Check sheet for the modelled part. Datum: model origin and axes. Units: mm. A direction names the side the tool comes from. Give positions to 0.01 mm unless a question says otherwise; leave off trailing zeros. Write each loop counter-clockwise with the first axis right and the second up, starting at its lowest first coordinate (ties: lowest second). Pieces come first, ordered by that corner, then holes. Notation, with made-up numbers: M 0.25,-2.75 L 16.25,-2.75 A6 cw 16.25,4.25 Z; hole C -27.75,-26 d5. An arc over 180 degrees is marked long. Write item = value, one per line. Start each with the question number.
1) Sectioned sample at D-D, the plane x = -0.5. Record the cut outline in (y, z), then the cut area to 3 significant figures.
2) Scan lines: L1, parallel to X at y = 3.5, z = -1.9; L2, parallel to Y at x = 3.5, z = 1.1; L3, parallel to X at y = -4.5, z = 1.75. Record each from-to range of solid material in increasing order.
3) Sectioned sample at B-B, the plane y = -3.75. Record the cut outline in (x, z), then the cut area to 3 significant figures.
4) Gauge pin test, flat ends, axial feed: pin 1 (0.5 mm diameter, centred on x = -2.5, z = 0.5, fed in from -Y); pin 2 (1.6 mm diameter, centred on x = -1.5, z = 1, fed in from +Y). Record the tip position at first contact, or that the pin passes through.
5) Sectioned sample at A-A, the plane x = 3.5. Record the cut outline in (y, z).
6) Sectioned sample at C-C, the plane z = 2.1. Record the cut outline in (x, y), then the cut area to 3 significant figures.
7) Draft check along X on faces 1 (the face through (5, -4, 0)), 2 (the face through (2, -7, 0)), 3 (the face through (0, 5, 0)), 4 (the face through (-3, 0, 0)). Enter one of: pulls with the +X half, pulls with the -X half, needs draft (parallel to the pull), parting line crosses it, or undercut.
8) Set-up check for faces 5 (the face through (-2.5, 4, 0)), 6 (the face through (-0.986, 2.048, -1.984)), 7 (the face through (-2.5, -4, 0)), 8 (the face through (4, -1, 0)): record each of +Z, -Z, +X, -X, +Y, -Y from which the full face is reachable in a straight line by a thin tool's end or side.
Autodesk Fusion 360 part; units mm, degrees
ref_plane "WorkPlane1" through (11.25, 0, 0) normal (1, 0, 0) x (0, 1, 0)
sketch "wire_screw2" plane through (0, 0, 0) normal (1, 0, 0) x (0, 1, 0)
  line L0 (7, 3.1) -> (-7, -3.1) construction
  line L1 (-7, 3.1) -> (7, -3.1) construction
  line L2 (-4, 4) -> (-4, -3.4897)
  line L3 (4, 4) -> (4, -3.5621)
  circle A0 centre (0, 0) radius 3.1
  circle A1 centre (0, 0) radius 2.75
  line L4 (-3.0288, -3.6864) -> (-3.0994, -0.0604)
  arc A2 (0, 2.75) -> (-3.0994, -0.0604) centre (0, -0.3643) ccw
  arc A3 (0, -2.75) -> (0, 2.75) centre (0, 0) ccw
  arc A4 (0, -2.75) -> (3.1, 0) centre (0, 0.3723) ccw
  line L5 (3.1, 0) -> (3.1, 3.8294)
  line L6 (0, 2.75) -> (3.1, 2.75)
  line L7 (0, -2.75) -> (-3.047, -2.75)
  line L8 (0, 2.75) -> (7, 2.75)
  line L9 (7, 2.75) -> (-7, 2.75)
  line L10 (-7, 2.75) -> (-7, -2.75)
  line L11 (-7, -2.75) -> (7, -2.75)
  line L12 (7, -2.75) -> (7, 2.75)
  dimension "d38" = 14
  dimension "d39" = 6.2
  dimension "d40" = 5.5
  dimension "d41" = 7
  dimension "d42" = 14
extrude "Extrude7" add sketch "wire_screw2" along normal blind -2 and the other way blind 3 contours L2 A0 L4 L9 L11 | A0 A2 L9 | A0 L4 L7 L11 | A0 L5 L6 L8 L9 | A0 A1 A3 A4 L6 L8 L9 | A0 A1 A2 L7 L11 | A1 A3 | L3 A0 L5 L8 L9 L11 | A0 A4 L11
extrude "Extrude8" add sketch "wire_screw2" against normal blind 2 contours A0 L4 L7 L11 | A0 L5 L6 L8 L9 | A0 A1 A3 A4 L6 L8 L9 | A0 A1 A2 L7 L11 | A1 A3
extrude "Extrude9" add sketch "wire_screw2" along normal blind 5 contours L2 A0 L4 L9 L11 | L2 L9 L10 L11 | A0 A2 L9 | A0 L4 L7 L11 | A0 L5 L6 L8 L9 | A0 A1 A3 A4 L6 L8 L9 | A0 A1 A2 L7 L11 | A1 A3 | L3 A0 L5 L8 L9 L11 | A0 A4 L11 | L3 L8 L9 L11 L12
sketch "wire_screw2_slot" plane through (0, 0, -2.75) normal (0, 0, -1) x (1, 0, 0)
  line L0 (-2, -4) -> (-2, 0)
  line L1 (-2, 0) -> (0, 0)
  line L2 (0, 0) -> (0, -7)
  line L3 (0, -7) -> (5, -7)
  line L4 (5, -7) -> (5, 7)
  line L5 (5, 7) -> (0, 7)
  line L6 (0, 7) -> (0, 3.047)
  line L7 (0, 3.047) -> (-2, 3.047)
  line L8 (-2, 3.047) -> (-2, 4)
  line L9 (-2, 4) -> (-3, 4)
  line L10 (-3, 4) -> (-3, -4)
  line L11 (-3, -4) -> (-2, -4)
  line L12 (3, 1) -> (7, 1)
  line L13 (7, 1) -> (7, -1)
  line L14 (7, -1) -> (3, -1)
  line L15 (3, -1) -> (3, 1)
  line L16 (3, 1) -> (7, -1) construction
  line L17 (7, 1) -> (3, -1) construction
  point P0 (5, 0)
  dimension "d51" = 4
  dimension "d52" = 2
extrude "Extrude10" cut sketch "wire_screw2_slot" against normal blind 8 contours L4 L12 L14 L15
Data:
q1.outline = M -3.1,-0.06 L -3.05,-2.75 L 0,-2.75 A3.12 ccw 3.1,0 L 3.1,2.75 L 0,2.75 A3.11 ccw Z
q1.area = 30.0 mm2
q2.L1 = -3 to -2, 0 to 5
q2.L2 = -7 to -1, 1 to 7
q2.L3 = 0 to 5
q3.outline = M -3,-2.75 L -2,-2.75 L -2,2.75 L -3,2.75 Z; M 0,-2.75 L 5,-2.75 L 5,2.75 L 0,2.75 Z
q3.area = 33.0 mm2
q4.pin_1 = -4
q4.pin_2 = 4
q5.outline = M -7,-2.75 L -1,-2.75 L -1,2.75 L -7,2.75 Z; M 1,-2.75 L 7,-2.75 L 7,2.75 L 1,2.75 Z
q6.outline = M -3,-4 L -2,-4 L -2,-1.9 L 0,-1.9 L 0,-7 L 5,-7 L 5,-1 L 3,-1 L 3,1 L 5,1 L 5,7 L 0,7 L 0,3.1 L -2,3.1 L -2,4 L -3,4 Z
q6.area = 84.0 mm2
q7.face_1 = pulls with the +X half
q7.face_2 = needs draft
q7.face_3 = undercut
q7.face_4 = pulls with the -X half
q8.face_5 = +Z, -Z, -X, +Y
q8.face_6 = -Z, +Y
q8.face_7 = +Z, -Z, -X, -Y
q8.face_8 = +Z, -Z, +X
